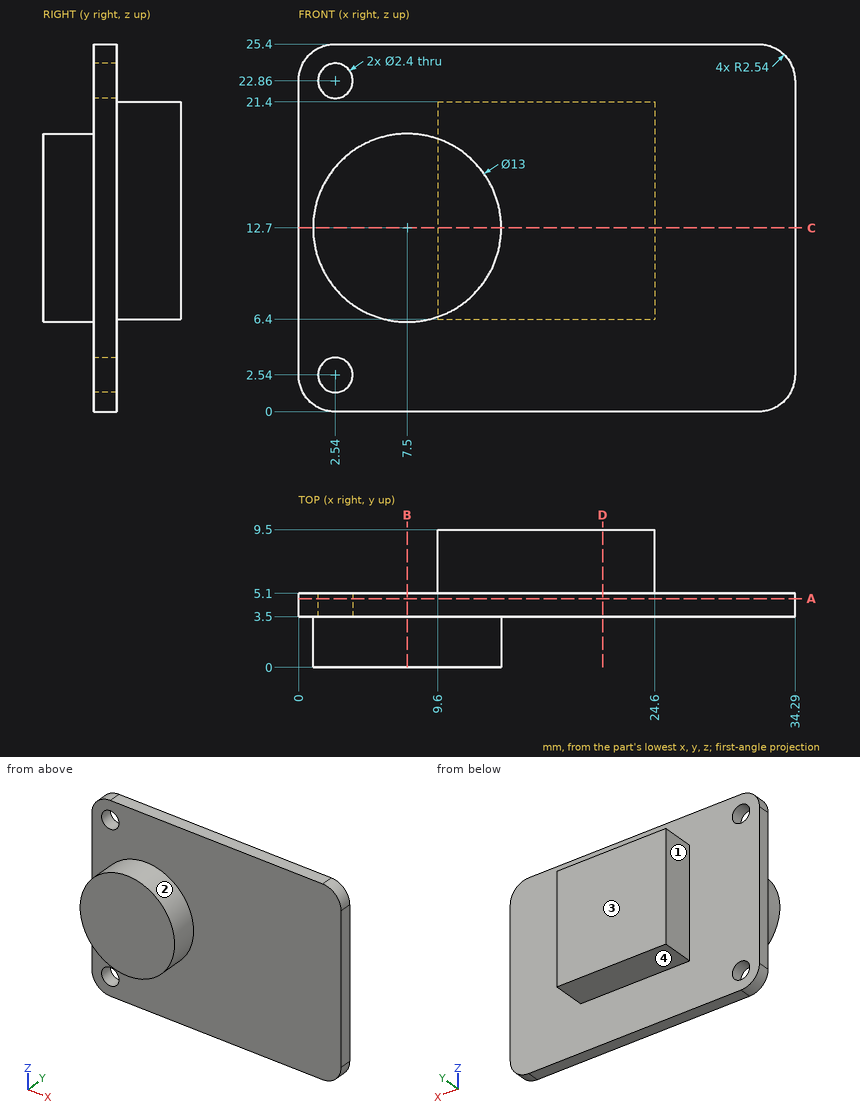
Input: dimensioned drawing with shaded views. Units: mm. Origin: part minimum x, y, z. A direction names the side the tool comes from. Round coordinates to 2 decimals unless told otherwise and drop trailing zeros. Loops run counter-clockwise (first coordinate to the right, second up) from the corner with the lowest first, then second, coordinate; pieces in that order, holes last. Notation, with made-up numbers: M -21,-28 L 27,-28 A28 cw 27,-3 Z; hole C -23,-39.75 d2. An arc over 180 degrees is marked long. One line per question, with ' | ' between items.
(1) Cut plane A-A on y = 4.75. Return the cut outline in (x, z).
Check result:
outline: M 0,2.54 A2.54 ccw 2.54,0 L 31.75,0 A2.54 ccw 34.29,2.54 L 34.29,22.86 A2.54 ccw 31.75,25.4 L 2.54,25.4 A2.54 ccw 0,22.86 Z; hole C 2.54,2.54 d2.4; hole C 2.54,22.86 d2.4
(2) Contact query for flat-ended pins moving along their axis: P1, Ø2, axis at x = 4.5, z = 8.5, coming from the +Y side; P2, Ø1.3, axis at x = 19, y = 7, coming from the -Z side; P3, Ø1.3, axis at x = 14.5, y = 7.5, coming from the +Z side. Output: stop coordinate, or through.
Check result:
P1: stops at y = 5.1 | P2: stops at z = 6.4 | P3: stops at z = 21.4
(3) Access query for the marked faces 1, 2, 3 and 4. Directions: +Z, -Z, +X, -X, +Y, -Y. A direction counts if a zero-diameter tool reaches every point of the face in a straight line with its end or side. Return the directions, or none.
Check result:
face 1: +Z, -Z, -X, +Y | face 2: -Y | face 3: +Z, -Z, +X, -X, +Y | face 4: -Z, +X, -X, +Y
(4) Cut plane B-B on x = 7.5. Return the cut outline in (y, z), plus the area to 3 significant figures.
Check result:
outline: M 0,6.2 L 3.5,6.2 L 3.5,0 L 5.1,0 L 5.1,25.4 L 3.5,25.4 L 3.5,19.2 L 0,19.2 Z | area: 86.1 mm2
(5) Cut plane D-D on x = 21. Return the cut outline in (y, z).
Check result:
outline: M 3.5,0 L 5.1,0 L 5.1,6.4 L 9.5,6.4 L 9.5,21.4 L 5.1,21.4 L 5.1,25.4 L 3.5,25.4 Z
(6) Material intervals for line 1 along Z through (x, y) = (2.54, 4.25); line 2 along X through (y, z) = (4.3, 22.86); line 3 along Y through (x, z) = (20, 14), sorted ascending. Write a range as from..to.
Check result:
line 1: z = 0..1.34, 3.74..21.66, 24.06..25.4 | line 2: x = 0..1.34, 3.74..34.29 | line 3: y = 3.5..9.5
(7) Cut plane C-C on z = 12.7. Return the cut outline in (x, y), plus the area to 3 significant figures.
Check result:
outline: M 0,3.5 L 1,3.5 L 1,0 L 14,0 L 14,3.5 L 34.29,3.5 L 34.29,5.1 L 24.6,5.1 L 24.6,9.5 L 9.6,9.5 L 9.6,5.1 L 0,5.1 Z | area: 166 mm2
